Read the model definition and answer for the solid it produces. Units are mm, in the model's axes. A direction names the side the tool comes from. Round coordinates to 2 decimals unless told otherwise and drop trailing zeros. Loops run counter-clockwise (first coordinate to the right, second up) from the corner with the lowest first, then second, coordinate; pieces in that order, holes last. Notation, with made-up numbers: (32, 65) - (37, 65) arc R20 cw to (37, 98) - close; hole circle Ø4 at (-30, 88). An arc over 180 degrees is marked (long way). Answer as CSV lines item,"result".
Autodesk Inventor part; units mm, degrees
ref_plane "Work Plane1" through (0, 0, -5) normal (0, 0, 1) x (1, 0, 0)
ref_plane "YZ Plane" through (0, 0, 0) normal (1, 0, 0) x (0, 1, 0)
ref_plane "XZ Plane" through (0, 0, 0) normal (0, 1, 0) x (-1, 0, 0)
sketch "Sketch1" plane through (0, 0, 0) normal (0, 1, 0) x (-1, 0, 0)
  circle A0 centre (0, 0) radius 5
  dimension "d0" = 10
extrude "Extrusion1" add sketch "Sketch1" along normal blind 32
sketch "Sketch2" plane through (0, 32, 0) normal (0, 1, 0) x (1, 0, 0)
  line L0 (-1.5, 5) -> (1.5, 5)
  line L1 (1.5, 5) -> (1.5, -5)
  line L2 (1.5, -5) -> (-1.5, -5)
  line L3 (-1.5, -5) -> (-1.5, 5)
  point P0 (0, 0)
  point P1 (-1.5, 0)
  point P2 (0, 5)
  dimension "d3" = 3
  dimension "d4" = 10
extrude "Extrusion2" cut sketch "Sketch2" against normal blind 8
sketch "Sketch3" plane through (1.5, 32, -4.7697) normal (-1, 0, 0) x (0, 0, 1)
  circle A0 centre (4.7697, -4) radius 1
  line L0 (9.5394, 0) -> (0, 0)
  point P0 (4.7697, -32)
  point P1 (4.7697, 0)
  dimension "d7" = 2
  dimension "d8" = 4
extrude "Extrusion3" add sketch "Sketch3" along normal blind 3
ref_plane "Work Plane1" through (0, 0, -5) normal (0, 0, 1) x (1, 0, 0)
sketch "Sketch5" plane through (0, 0, -5) normal (0, 0, 1) x (1, 0, 0)
  point P0 (0, 0)
  point P1 (0, 7)
  dimension "d14" = 7
hole "Hole1" at (0, 7, -5) direction (0, 0, 1) diameter 3.302 end through all countersink diameter 8 countersink angle 90
chamfer "Chamfer1" distance 2 angle 45 1 edges at (-0.2563, 5.369, 4.9934)
equation "\"d20\" = Thickness"
equation "\"BendRadius\" = Thickness"
equation "\"BendReliefWidth\" = Thickness"
equation "\"BendReliefDepth\" = 0.5 * Thickness"
equation "\"CornerReliefSize\" = 4 * Thickness"
equation "\"MinimumRemnant\" = 2 * Thickness"
equation "\"TransitionRadius\" = BendRadius"
equation "\"GapSize\" = Thickness"
properties part number "barrel_hinge-female" material "Stainless Steel"
1) The mould has two halves that part along Y. Classify faces 1 (the face through (1.6, 6.6, 0.2)), 2 (the face through (0, 0, 0)), 3 (the face through (3, 32, 0)): pulls with the +Y half, pulls with the -Y half, needs draft (parallel to the pull), parting line crosses it, or undercut.
Entries:
face 1,"undercut"
face 2,"pulls with the -Y half"
face 3,"pulls with the +Y half"
2) A cutting plane is placed at A-A, the plane z = 0. Determine the outline of the cut face in (x, y), plus the area to 3 significant figures.
Entries:
outline,"(-5, 0) - (5, 0) - (5, 32) - (1.5, 32) - (1.5, 29) - (-1.5, 29) - (-1.5, 32) - (-5, 32) - close; hole circle Ø3.3 at (0, 7); hole (-1.5, 24) - (1.5, 24) - (1.5, 27) - (-1.5, 27) - close"
area,"293 mm^2"
3) A tool of negligible diameter and unlimited length cuts with its end or side. For faces 4 (the face through (0, 27, 0)), 5 (the face through (-3, 32, 0)), from which of +Z, -Z, +X, -X, +Y, -Y can it reach the whole face along a straight path? Write none if from no direction.
Entries:
face 4,"none"
face 5,"+Z, -Z, +X, -X, +Y"
4) Each of these flat-tipped pins is pushed along its axis until it touches: P1, Ø1.5, axis at y = 26, z = 2, coming from the -X side; P2, Ø0.9, axis at x = 0.5, z = 2.5, coming from the +Y side; P3, Ø4, axis at x = 0, y = 7, coming from the -Z side. Where does it stop, or does it pass through?
Entries:
P1,"stops at x = -4.84"
P2,"stops at y = 24"
P3,"stops at z = -3"
5) A cutting plane is placed at B-B, the plane x = 0. Count the separate pieces of the cut face and the enclosed holes in it, plus the area to 3 significant figures.
Entries:
separate pieces,"3"
enclosed holes,"0"
area,"201 mm^2"
6) A cutting plane is placed at C-C, the plane y = 28. Determine the outline of the cut face in (x, z), plus the area to 3 significant figures.
Entries:
outline,"(-1.5, -4.77) - (-1.5, -1) - (1.5, -1) - (1.5, -4.77) arc R5 ccw to (1.5, 4.77) - (1.5, 1) - (-1.5, 1) - (-1.5, 4.77) arc R5 ccw to start"
area,"55.0 mm^2"
7) Find the intervals of material crossed by line 1 (Y direction, x = 0, z = 0); line 2 (X direction, y = 7, z = 0.2); line 3 (Y direction, x = 0, z = 0.65), in increasing order.
Entries:
line 1,"y = 0 to 5.35, 8.65 to 24, 27 to 29"
line 2,"x = -5 to -1.65, 1.65 to 5"
line 3,"y = 0 to 5.35, 8.65 to 24, 27.24 to 28.76"
8) A cutting plane is placed at D-D, the plane z = -1.75. Determine the outline of the cut face in (x, y).
Entries:
outline,"(-4.68, 0) - (4.68, 0) - (4.68, 32) - (1.5, 32) - (1.5, 24) - (-1.5, 24) - (-1.5, 32) - (-4.68, 32) - close; hole circle Ø3.3 at (0, 7)"
